Input: part model. Units: mm. Frame: model coordinates. Face numbers are marked on the shaded views. A direction names the side the tool comes from. Give positions to 0.01 mm unless a question says otherwise; leave off trailing zeros. Write each loop counter-clockwise with the first axis right and the second up, starting at its lowest first coordinate (ties: lowest second). Pieces come first, ordered by that corner, then holes. Notation, with made-up numbers: (66, 71) -> (76, 71) arc R7 ccw to (76, 77) -> close; hole circle Ø1 at (47.25, 60). An arc over 180 degrees is marked (long way). Return JSON: item names as keys, results as strings. Group by question number.
Item 1: Section B-B, the plane x = -1. Count the separate pieces of the cut face and the enclosed holes in it, then the cut area to 3 significant figures.
Item 2: Section A-A, the plane y = -0.75. Return loops of the section in (x, z).
Item 3: Section D-D, the plane y = -4. Return loops of the section in (x, z), then the cut area to 3 significant figures.
Item 4: Mould query, pull axis X, two halves, no side actions, for the marked faces 1, 2 and 3. Classes: released by +X, released by -X, zero draft, split by the parting line, or undercut.
Item 5: Line query: line 1 (Y direction, x = 13, z = 48.25); line 2 (X direction, y = -8, z = 50.25); line 3 (X direction, y = -4.5, z = 49). Output: solid intervals per line, ascending. Write a range as [from, to].
Item 6: Pin query (flat end, axial travel): P1, Ø3.5, axis at x = -1.5, z = 47.5, coming from the -Y side; P2, Ø2.5, axis at x = 10.5, y = -5.5, coming from the -Z side; P3, Ø1.5, axis at y = 3, z = 48.5, coming from the +X side. Return the tip coordinate at first contact, or that it passes through.
Item 7: Section C-C, the plane z = 49.25. Return loops of the section in (x, y), then the cut area to 3 significant figures.
Item 8: Set-up query: the marked faces 4, 5, 6, 7 and 8. Return all of +Z, -Z, +X, -X, +Y, -Y with unobstructed straight access to the full face (end or side cutting, diameter ignored); none if empty.
from build123d import *

# Parameters (mm, degrees)
SKETCH025_W       = 36.5
SKETCH025_H       = 19
PAD016_DEPTH      = 3
THICKNESS004_T    = 1
SKETCH026_W       = 36.5
SKETCH026_H       = 19
SKETCH026_W_2     = 34.5
SKETCH026_H_2     = 18
PAD017_DEPTH      = 3
PAD017_DEPTH_BACK = 5
FILLET005_R       = 1
POCKET007_DEPTH   = 1
CHAMFER002_SIZE   = 0.49


with BuildPart() as part:
    # Sketch025 → Pad016 (new body)
    with BuildSketch(Plane.XY):
        Rectangle(SKETCH025_W, SKETCH025_H)
    extrude(amount=PAD016_DEPTH)

    # Thickness004
    thickness004_openings = [part.faces().sort_by_distance(p)[0] for p in [
        (0, 0, 0),
    ]]
    offset(amount=THICKNESS004_T, openings=thickness004_openings)

    # Sketch026 → Pad017 (join, two sides)
    with BuildSketch(Plane.XY) as pad017_sk:
        Rectangle(SKETCH026_W, SKETCH026_H)
        Rectangle(SKETCH026_W_2, SKETCH026_H_2, mode=Mode.SUBTRACT)
    extrude(amount=PAD017_DEPTH)
    extrude(pad017_sk.sketch, amount=-PAD017_DEPTH_BACK)

    # Fillet005
    fillet005_edges = [part.edges().sort_by_distance(p)[0] for p in [
        (18.25, -9.5, -2.5),
        (18.25, 9.5, -2.5),
        (-18.25, 9.5, -2.5),
        (-18.25, -9.5, -2.5),
        (0, -9, 3),
        (17.25, 0, 3),
        (0, 9, 3),
        (-17.25, 0, 3),
    ]]
    fillet(fillet005_edges, radius=FILLET005_R)

    # Sketch031 → Pocket007 (cut)
    with BuildSketch(Plane.XY):
        Polygon((-28.138837, 2.5), (-2.5, 2.5), (-2.5, 15.913807), (2.5, 15.913807), (2.5, 2.5), (28.138837, 2.5), (28.138837, -2.5), (2.5, -2.5), (2.5, -15.913807), (-2.5, -15.913807), (-2.5, -2.5), (-28.138837, -2.5), align=None)
    extrude(amount=POCKET007_DEPTH, mode=Mode.SUBTRACT)

    # Chamfer002
    chamfer002_edges = [part.edges().sort_by_distance(p)[0] for p in [
        (-18.25, 0, -5),
        (18.25, 0, -5),
    ]]
    chamfer(chamfer002_edges, length=CHAMFER002_SIZE)


with BuildPart() as part_1:
    # Body006 placement: moved
    add(part.part.moved(Location((0, 0, 50))))


solid = part_1.part
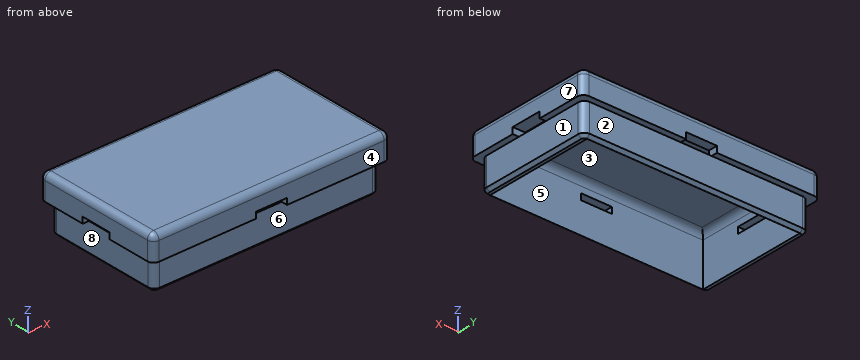
Answer below:
{
 "1": {"separate pieces": "3", "enclosed holes": "0", "area": "31.8 mm2"},
 "2": {"outline": "(-19.25, 51) -> (-17.25, 51) -> (-17.25, 52) arc R1 cw to (-16.25, 53) -> (16.25, 53) arc R1 cw to (17.25, 52) -> (17.25, 51) -> (19.25, 51) -> (19.25, 53) arc R1 ccw to (18.25, 54) -> (-18.25, 54) arc R1 ccw to (-19.25, 53) -> close; (-18.25, 45.49) -> (-17.76, 45) -> (-17.25, 45) -> (-17.25, 50) -> (-18.25, 50) -> close; (17.25, 45) -> (17.76, 45) -> (18.25, 45.49) -> (18.25, 50) -> (17.25, 50) -> close"},
 "3": {"outline": "(-19.25, 50) -> (-18.25, 50) -> (-18.25, 45.49) -> (-17.76, 45) -> (-17.25, 45) -> (-17.25, 52) arc R1 cw to (-16.25, 53) -> (16.25, 53) arc R1 cw to (17.25, 52) -> (17.25, 45) -> (17.76, 45) -> (18.25, 45.49) -> (18.25, 50) -> (19.25, 50) -> (19.25, 53) arc R1 ccw to (18.25, 54) -> (-18.25, 54) arc R1 ccw to (-19.25, 53) -> close", "area": "60.3 mm2"},
 "4": {"face 1": "released by +X", "face 2": "zero draft", "face 3": "undercut"},
 "5": {"line 1": "y = [-9.5, -9], [9, 9.5]", "line 2": "x = [-19.25, -17.25], [17.25, 19.25]", "line 3": "x = [-18.25, -17.25], [17.25, 18.25]"},
 "6": {"P1": "stops at y = -9.5", "P2": "stops at z = 53", "P3": "stops at x = 18.25"},
 "7": {"outline": "(-18.25, -8.5) arc R1 ccw to (-17.25, -9.5) -> (17.25, -9.5) arc R1 ccw to (18.25, -8.5) -> (18.25, 8.5) arc R1 ccw to (17.25, 9.5) -> (-17.25, 9.5) arc R1 ccw to (-18.25, 8.5) -> close; hole (-17.25, -9) -> (17.25, -9) -> (17.25, 9) -> (-17.25, 9) -> close", "area": "71.6 mm2"},
 "8": {"face 4": "+Z, -Z, +X, -X, -Y", "face 5": "-Z", "face 6": "-Z, +X, -X, -Y", "face 7": "+Z, -Z, +X, +Y, -Y", "face 8": "-Z, -X, +Y, -Y"}
}
